Geometry: final body of the model. Coordinates: model frame, mm. Round coordinates to 2 decimals unless told otherwise and drop trailing zeros. Loops run counter-clockwise (first coordinate to the right, second up) from the corner with the lowest first, then second, coordinate; pieces in that order, holes last. Notation, with made-up numbers: (86.5, 35) - (91.5, 35) arc R5 cw to (91.5, 39) - close; hole circle Ø4 at (43.5, 27). An arc over 180 degrees is marked (long way). Use CSV: the item, a comma, the result in double quotes.
from build123d import *

# Parameters (mm, degrees)
SKETCH1_R    = 1.2319
RODEND_DEPTH = 40.64
SKETCH2_W    = 6.35
SKETCH2_H    = 2.4638
SKETCH2_W_2  = 2.4638
SKETCH2_H_2  = 1.524
FLATS_DEPTH  = 5.715
SKETCH3_R    = 0.5715
HOLE_DEPTH   = 41.707527741
SKETCH4_R    = 1.2319
REV1_ANGLE   = 70
SKETCH6_R    = 1.2319
REV2_ANGLE   = 70
SKETCH10_R   = 1.2319
SHAFT_DEPTH  = 152.4


with BuildPart() as part:
    # Sketch1 → RodEnd (new body)
    with BuildSketch(Plane.XY):
        Circle(SKETCH1_R)
    extrude(amount=-RODEND_DEPTH)

    # Sketch2 → Flats (cut)
    with BuildSketch(Plane.XY):
        Rectangle(SKETCH2_W, SKETCH2_H)
        Rectangle(SKETCH2_W_2, SKETCH2_H_2, mode=Mode.SUBTRACT)
    extrude(amount=-FLATS_DEPTH, mode=Mode.SUBTRACT)

    # Sketch3 → Hole (cut, through all)
    with BuildSketch(Plane(origin=(0, 0.762, 0), x_dir=(1, 0, 0), z_dir=(0, 1, 0))):
        with Locations(Location((0, 1.27, 0), (0, 0, 270))):
            Circle(SKETCH3_R)
    extrude(amount=-HOLE_DEPTH, mode=Mode.SUBTRACT)

    # Sketch4 → Rev1 (revolve)
    with BuildSketch(Plane(origin=(0, 0, -40.64), x_dir=(-1, 0, 0), z_dir=(0, 0, -1))):
        with Locations(Location((0, 0, 0), (0, 0, 180))):
            Circle(SKETCH4_R)
    revolve(axis=Axis((-1.27, 0, -40.64), (0, 1, 0)), revolution_arc=REV1_ANGLE)

    # Sketch6 → Rev2 (revolve)
    with BuildSketch(Plane(origin=(-14.18288245, 0, -5.162147048), x_dir=(-0.3420201433256661, 0, 0.9396926207859093), z_dir=(-0.9396926207859094, 0, -0.34202014332566616))):
        with Locations((-39.024742527, 0)):
            Circle(SKETCH6_R)
    revolve(axis=Axis((-0.401268836, 0, -43.026819257), (0, -1, 0)), revolution_arc=REV2_ANGLE)

    # Sketch10 → Shaft (add)
    with BuildSketch(Plane(origin=(0, 0, -43.026819257), x_dir=(-1, 0, 0), z_dir=(0, 0, -1))):
        with Locations((1.671268836, 0)):
            Circle(SKETCH10_R)
    extrude(amount=SHAFT_DEPTH)


solid = part.part
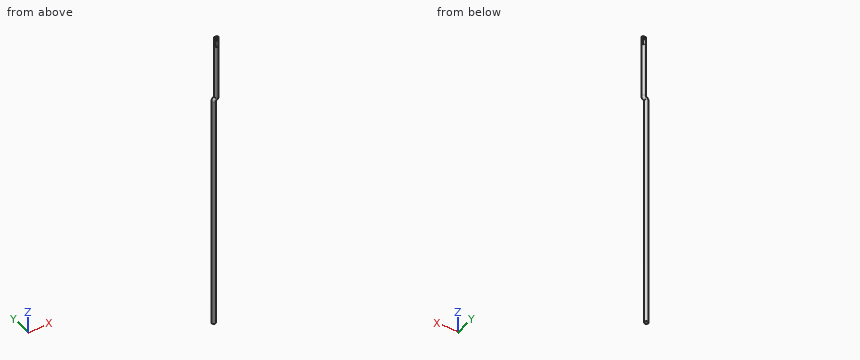
Item 1: Pin query (flat end, axial travel): P1, Ø0.9, axis at x = 0, z = -1.27, coming from the -Y side; P2, Ø1, axis at y = 0.5, z = -32.5, coming from the +X side; P3, Ø2, axis at x = 0, z = -2, coming from the +Y side; P4, Ø1.5, axis at x = -0.5, z = -2, coming from the -Y side. Return the tip coordinate at first contact, or that it passes through.
Final values:
P1,"passes through"
P2,"stops at x = 1.23"
P3,"stops at y = 0.76"
P4,"stops at y = -0.76"
Item 2: Section B-B on z = -58. Return the cut outline in (x, y), plus the area to 3 significant figures.
Final values:
outline,"circle Ø2.46 at (-1.67, 0)"
area,"4.77 mm²"
Item 3: Section A-A on y = 0. Return the cut outline in (x, z).
Final values:
outline,"(-2.9, -195.43) - (-0.44, -195.43) - (-0.44, -43.03) arc R0.04 cw to (-0.41, -42.99) arc R2.5 ccw to (1.23, -40.64) - (1.23, 0) - (-1.23, 0) - (-1.23, -40.64) arc R0.04 cw to (-1.26, -40.68) arc R2.5 ccw to (-2.9, -43.03) - close; hole circle Ø1.14 at (0, -1.27)"
Item 4: Material intervals for line 1 (X direction, y = -0.2, z = -1.27); line 2 (X direction, y = -0.3, z = -89); line 3 (X direction, y = -0.05, z = -90), sorted ascending.
Final values:
line 1,"x = -1.22 to -0.57, 0.57 to 1.22"
line 2,"x = -2.87 to -0.48"
line 3,"x = -2.9 to -0.44"
